Source: three-view drawing plus pictorial views. Frame: mm from the lowest corner of the part. A direction names the side the tool comes from. Round coordinates to 2 decimals unless told otherwise and drop trailing zeros. Order: outer loops, then holes, each group sorted by start corner. A loop starts at its lowest first (then second) coordinate and runs counter-clockwise, first axis right, second up. Notation, with made-up numbers: (-2.75, 31.5) -> (41.25, 31.5) arc R24 ccw to (41.25, 49.5) -> close; hole circle Ø3 at (66, 36.25). An arc over 180 degrees is marked (long way). Use a Markdown table: item, result.
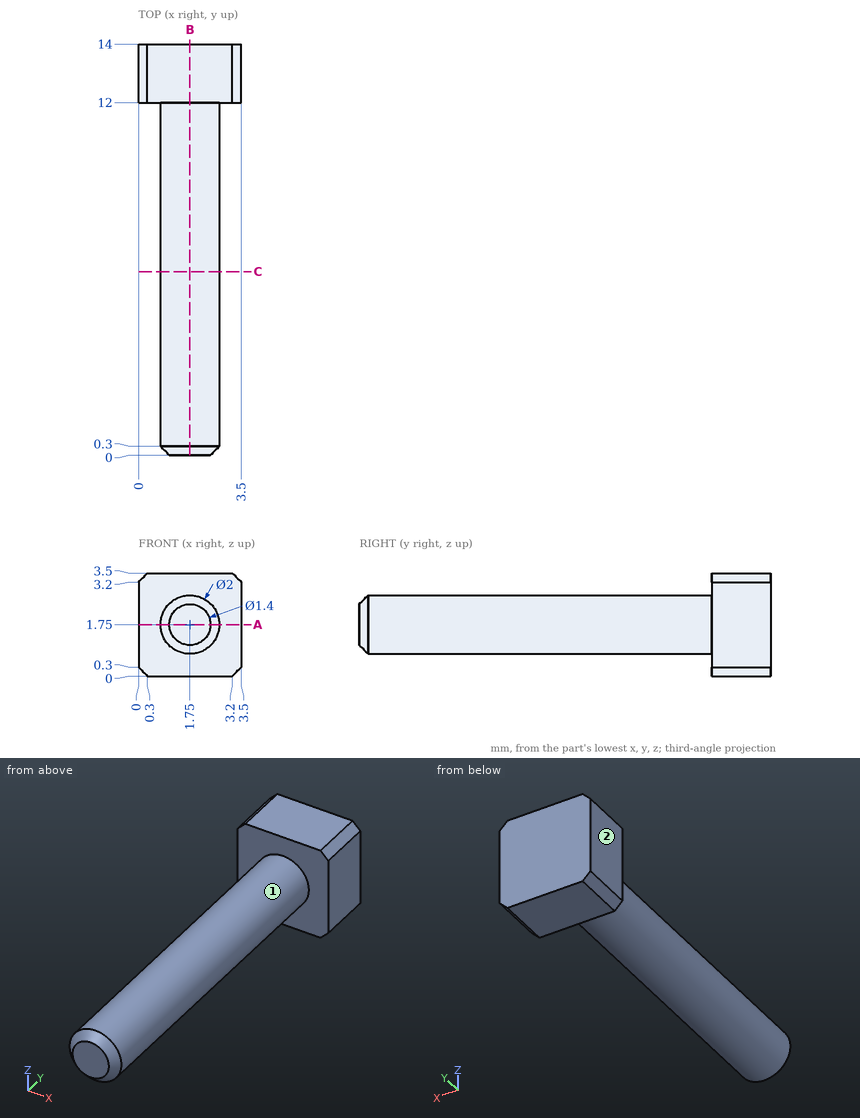
1) Cut plane A-A on z = 1.75. Return loops of the section in (x, y), and give its area (3 significant figures).
Results found:
| item | result |
|---|---|
| outline | (0, 12) -> (0.75, 12) -> (0.75, 0.3) -> (1.05, 0) -> (2.45, 0) -> (2.75, 0.3) -> (2.75, 12) -> (3.5, 12) -> (3.5, 14) -> (0, 14) -> close |
| area | 30.9 mm² |
2) Line query: L1, parallel to Y at x = 3.2, z = 0.2; L2, parallel to X at y = 7.5, z = 1.85; L3, parallel to Y at x = 0.8, z = 1.6. Output: solid intervals per line, ascending. Write a range as [from, to].
Results found:
| item | result |
|---|---|
| L1 | y = [12, 14] |
| L2 | x = [0.76, 2.74] |
| L3 | y = [0.26, 14] |
3) Cut plane C-C on y = 6.25. Return loops of the section in (x, z), and give its area (3 significant figures).
Results found:
| item | result |
|---|---|
| outline | circle Ø2 at (1.75, 1.75) |
| area | 3.14 mm² |
4) Cut plane B-B on x = 1.75. Return loops of the section in (y, z).
Results found:
| item | result |
|---|---|
| outline | (0, 1.05) -> (0.3, 0.75) -> (12, 0.75) -> (12, 0) -> (14, 0) -> (14, 3.5) -> (12, 3.5) -> (12, 2.75) -> (0.3, 2.75) -> (0, 2.45) -> close |
5) Set-up query: the marked faces 1 and 2. Return all of +Z, -Z, +X, -X, +Y, -Y with unobstructed straight access to the full face (end or side cutting, diameter ignored); none if empty.
Results found:
| item | result |
|---|---|
| face 1 | -Y |
| face 2 | +Z, -Z, -X, +Y, -Y |
6) Pin query (flat end, axial travel): pin 1 Ø1 at (x, y) = (2, 7) entering from -Z; pin 2 Ø2 at (x, y) = (2, 4) entering from +Z. Return the tip coordinate at first contact, or that it passes through.
Results found:
| item | result |
|---|---|
| pin 1 | stops at z = 0.75 |
| pin 2 | stops at z = 2.75 |
